Build history of the part. All positions in model axes, mm. Face numbers are marked on the shaded views. A direction names the side the tool comes from. Give positions to 0.01 mm unless a question says otherwise; leave off trailing zeros. Order: outer loops, then holes, each group sorted by start corner. A loop starts at its lowest first (then second) coordinate and runs counter-clockwise, first axis right, second up. Notation, with made-up numbers: (-3.75, 35.25) - (19.25, 35.25) arc R10 ccw to (19.25, 54.25) - close; hole circle Ø7 at (53.25, 38). An arc over 180 degrees is marked (long way). Use a Markdown table: item, result. Add a question column.
(1) Flat gauge pins, fed straight in: pin 1 (13 mm diameter, centred on x = -15, z = 21, fed in from -Y); pin 2 (6.5 mm diameter, centred on x = -20, z = 15, fed in from -Y); pin 3 (2.5 mm diameter, centred on x = -20, z = 15, fed in from -Y). Where does each tip first touch, or does it go through?
(2) Slice it at D-D (z = 26.5). Write the cut outline in (x, y), then the cut area to 3 significant figures.
(3) Slice it at C-C (x = -20). Write the cut outline in (y, z).
(4) Slice it at A-A (z = 15). Write the cut outline in (x, y).
(5) Which spindle directions (+Z, -Z, +X, -X, +Y, -Y) get a long thin tool onto all of the face, cutting with end or side? Do the marked faces 1 and 2. Say none if no direction does.
(6) Mould opens along Z. For the marked faces 3, 4 and 5 say: +Z half, -Z half, draft (parallel to the pull), parting line (faces both ways), or undercut.
(7) Slice it at B-B (y = 3.25). Write the cut outline in (x, z), then the cut area to 3 significant figures.
(8) Wall check: line 1 (Z direction, x = -20, y = 4.9); line 2 (Z direction, x = -20, y = 3.05); line 3 (Y direction, x = -5, z = 7). Give the ranges that are in metal, low to high.
from build123d import *

# Parameters (mm, degrees)
F1_DEPTH       = 6
F2_DEPTH       = 2
F3_D           = 4.2
F3_DEPTH       = 15
F3_CBORE_D     = 7
F3_CBORE_DEPTH = 4
F4_R           = 2


with BuildPart() as f1:
    # F0 (on Front) → F1 (new body)
    with BuildSketch(Plane.XZ):
        Polygon((-40, 0), (0, 0), (0, 30), (-40, 30), (-40, 15), align=None)
        Polygon((-38, 2), (-38, 15), (-38, 28), (-2, 28), (-2, 2), align=None, mode=Mode.SUBTRACT)
        Polygon((-38, 28), (-38, 15), (-38, 2), (-2, 2), (-2, 28), align=None)
    extrude(amount=-F1_DEPTH)

    # F0 (on Front) → F2 (join)
    with BuildSketch(Plane.XZ):
        Polygon((-40, 0), (0, 0), (0, 30), (-40, 30), (-40, 15), align=None)
        Polygon((-38, 2), (-38, 15), (-38, 28), (-2, 28), (-2, 2), align=None, mode=Mode.SUBTRACT)
    extrude(amount=F2_DEPTH)

    # F3
    with Locations(Plane.XZ):
        with Locations((-20, 15)):
            CounterBoreHole(F3_D / 2, F3_CBORE_D / 2, F3_CBORE_DEPTH, depth=F3_DEPTH)

    # F4
    f4_edges = [f1.edges().sort_by_distance(p)[0] for p in [
        (-40, 2, 30),
        (0, 2, 30),
        (0, 2, 0),
        (-40, 2, 0),
    ]]
    fillet(f4_edges, radius=F4_R)


solid = f1.part
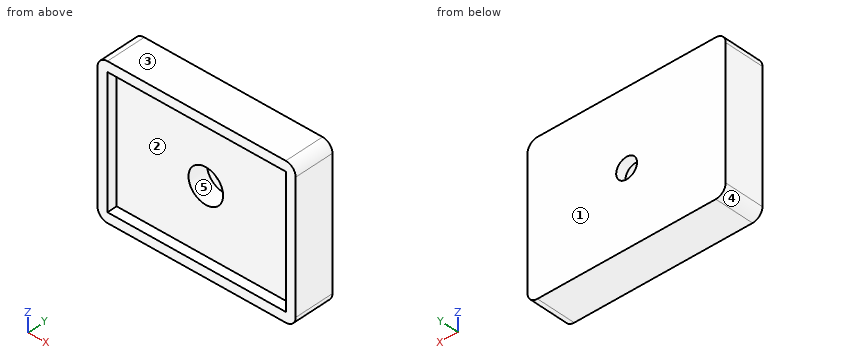
Solution:
| question | item | result |
|---|---|---|
| 1 | pin 1 | y = 0 |
| 1 | pin 2 | y = 4 |
| 1 | pin 3 | through |
| 2 | outline | (-40, -2) - (-38, -2) - (-38, 0) - (-2, 0) - (-2, -2) - (0, -2) - (0, 6) - (-40, 6) - close |
| 2 | area | 248 mm2 |
| 3 | outline | (-2, 0) - (6, 0) - (6, 12.9) - (4, 12.9) - (4, 11.5) - (0, 11.5) - (0, 2) - (-2, 2) - close; (-2, 28) - (0, 28) - (0, 18.5) - (4, 18.5) - (4, 17.1) - (6, 17.1) - (6, 30) - (-2, 30) - close |
| 4 | outline | (-40, -2) - (-38, -2) - (-38, 0) - (-23.5, 0) - (-23.5, 4) - (-22.1, 4) - (-22.1, 6) - (-40, 6) - close; (-17.9, 4) - (-16.5, 4) - (-16.5, 0) - (-2, 0) - (-2, -2) - (0, -2) - (0, 6) - (-17.9, 6) - close |
| 5 | face 1 | +Z, -Z, +X, -X, +Y |
| 5 | face 2 | -Y |
| 6 | face 3 | +Z half |
| 6 | face 4 | -Z half |
| 6 | face 5 | undercut |
| 7 | outline | (-40, 2) arc R2 ccw to (-38, 0) - (-2, 0) arc R2 ccw to (0, 2) - (0, 28) arc R2 ccw to (-2, 30) - (-38, 30) arc R2 ccw to (-40, 28) - close; hole circle Ø7 at (-20, 15) |
| 7 | area | 1,160 mm2 |
| 8 | line 1 | 0 to 12.9, 17.1 to 30 |
| 8 | line 2 | 0 to 11.5, 18.5 to 30 |
| 8 | line 3 | 0 to 6 |
